```python
from build123d import *

# Parameters (mm, degrees)
F0_R     = 2.9972
F1_DEPTH = 8.255
F0_R_2   = 4.0005
F2_DEPTH = 2.54
F3_R     = 1.9939
F4_DEPTH = 15.5448
F5_R     = 0.508
F6_R     = 0.762


with BuildPart() as f1:
    # F0 (on Front) → F1 (new body)
    with BuildSketch(Plane.XZ):
        Circle(F0_R)
    extrude(amount=-F1_DEPTH)

    # F0 (on Front) → F2 (join)
    with BuildSketch(Plane.XZ):
        Circle(F0_R_2)
        Circle(F0_R, mode=Mode.SUBTRACT)
    extrude(amount=-F2_DEPTH)

    # F3 (on Front) → F4 (join)
    with BuildSketch(Plane.XZ):
        Circle(F3_R)
    extrude(amount=-F4_DEPTH)

    # F5
    f5_edges = [f1.edges().sort_by_distance(p)[0] for p in [
        (-1.9939, 15.5448, 0),
    ]]
    fillet(f5_edges, radius=F5_R)

    # F6
    f6_edges = [f1.edges().sort_by_distance(p)[0] for p in [
        (-4.0005, 0, 0),
    ]]
    fillet(f6_edges, radius=F6_R)


solid = f1.part
```
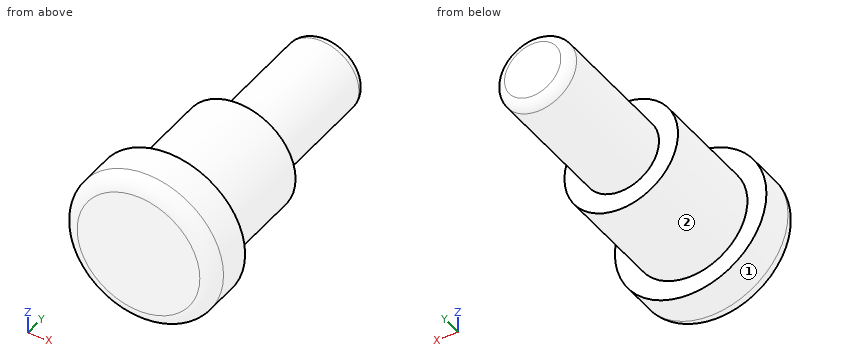
Could you check a few things on this model? Use its own coordinates, in mm. Face numbers are marked on the shaded views. A direction names the side the tool comes from. Round coordinates to 2 decimals unless told otherwise and drop trailing zeros. Loops run counter-clockwise (first coordinate to the right, second up) from the corner with the lowest first, then second, coordinate; pieces in that order, holes last. Notation, with made-up numbers: (59, 41.25) -> (78, 41.25) arc R24 cw to (78, 66.25) -> close; hole circle Ø5 at (50, 28). An arc over 180 degrees is marked (long way). Put each result on its own line as item: value.
Q1. I want a section at C-C on y = 11.75. Write out the boundary of the cut face in (x, z).
Checks:
outline: circle Ø3.99 at (0, 0)
Q2. I want a section at B-B on x = 0. Write out the boundary of the cut face in (y, z) (1 decimal).
Checks:
outline: (0, -3.2) arc R0.8 ccw to (0.8, -4) -> (2.5, -4) -> (2.5, -3) -> (8.3, -3) -> (8.3, -2) -> (15, -2) arc R0.5 ccw to (15.5, -1.5) -> (15.5, 1.5) arc R0.5 ccw to (15, 2) -> (8.3, 2) -> (8.3, 3) -> (2.5, 3) -> (2.5, 4) -> (0.8, 4) arc R0.8 ccw to (0, 3.2) -> close
Q3. I want a section at A-A on z = 0. Write out the boundary of the cut face in (x, y) (1 decimal), and give its area (3 significant figures).
Checks:
outline: (-4, 0.8) arc R0.8 ccw to (-3.2, 0) -> (3.2, 0) arc R0.8 ccw to (4, 0.8) -> (4, 2.5) -> (3, 2.5) -> (3, 8.3) -> (2, 8.3) -> (2, 15) arc R0.5 ccw to (1.5, 15.5) -> (-1.5, 15.5) arc R0.5 ccw to (-2, 15) -> (-2, 8.3) -> (-3, 8.3) -> (-3, 2.5) -> (-4, 2.5) -> close
area: 83.3 mm2
Q4. Please list where these lines run through material, in increasing order: line 1 (Y direction, x = 0, z = -2.75) (3 decimals); line 2 (Z direction, x = 0, y = 11.5); line 3 (Y direction, x = -3, z = 0.5). Write a range as from..to.
Checks:
line 1: 0..8.255
line 2: -1.99..1.99
line 3: 0..2.54
Q5. For pin 1 Ø1 at (y, z) = (5, -2) entering from -X; pin 2 Ø4 at (x, y) = (-0.5, 10) entering from -Z; pin 3 Ø3 at (y, z) = (12, -2) entering from +X, each with a flat end and sliding along its axis, tell me the tip position at first contact or that it passes through.
Checks:
pin 1: x = -2.59
pin 2: z = -3
pin 3: x = 1.93
Q6. Which directions (+Z, -Z, +X, -X, +Y, -Y) give clear straight access to the entire face, cutting with the end or side of a thin tool? Please do the marked faces 1 and 2.
Checks:
face 1: +Y, -Y
face 2: +Y
